The listing builds one solid part. Answer for the finished solid, in the listing's coordinates (mm). A direction names the side the tool comes from. Give positions to 0.01 mm unless a question says otherwise; leave off trailing zeros. Write each loop counter-clockwise with the first axis right and the second up, starting at its lowest first coordinate (ties: lowest second). Pieces come first, ordered by that corner, then holes. Notation, with made-up numbers: (65.25, 71.25) - (73.25, 71.25) arc R22 ccw to (73.25, 97.25) - close; hole circle Ø7 at (-35, 45). An arc over 180 degrees is marked (long way). Use a Markdown table: item, result. Add a question column.
from build123d import *

# Parameters (mm, degrees)
SKETCH1_W           = 12.7
SKETCH1_H           = 25.4
BOSS_EXTRUDE1_DEPTH = 3.175
SKETCH2_W           = 12.7
SKETCH2_H           = 3.175
BOSS_EXTRUDE2_DEPTH = 13.7922
SKETCH3_R           = 2.54
CUT_EXTRUDE1_DEPTH  = 4.175
CUT_EXTRUDE2_DEPTH  = 4.175
SKETCH5_R           = 2.54
CUT_EXTRUDE3_DEPTH  = 4.175
CUT_EXTRUDE4_DEPTH  = 4.175


with BuildPart() as part:
    # Sketch1 → Boss-Extrude1 (new body)
    with BuildSketch(Plane(origin=(0, 0, 0), x_dir=(1, 0, 0), z_dir=(0, 1, 0))):
        with Locations((-19.111794294, -7.819421488)):
            Rectangle(SKETCH1_W, SKETCH1_H)
    extrude(amount=BOSS_EXTRUDE1_DEPTH)

    # Sketch2 → Boss-Extrude2 (add)
    with BuildSketch(Plane(origin=(0, 3.175, 0), x_dir=(1, 0, 0), z_dir=(0, 1, 0))):
        with Locations((-19.111794294, -18.931921488)):
            Rectangle(SKETCH2_W, SKETCH2_H)
    extrude(amount=BOSS_EXTRUDE2_DEPTH)

    # Sketch3 → Cut-Extrude1 (cut, through all)
    with BuildSketch(Plane(origin=(0, 3.175, 0), x_dir=(1, 0, 0), z_dir=(0, 1, 0))):
        with Locations((-19.111794294, -2.739421488)):
            Circle(SKETCH3_R)
    extrude(amount=-CUT_EXTRUDE1_DEPTH, mode=Mode.SUBTRACT)

    # Sketch4 → Cut-Extrude2 (cut, through all)
    with BuildSketch(Plane(origin=(0, 3.175, 0), x_dir=(1, 0, 0), z_dir=(0, 1, 0))):
        with BuildLine():
            Line((-25.461794294, 4.880578512), (-12.761794294, 4.880578512))
            Line((-12.761794294, 4.880578512), (-12.761794294, 1.385127101))
            ThreePointArc((-12.761794294, 1.385127101), (-19.111794294, 4.832526813), (-25.461794294, 1.385127101))
            Line((-25.461794294, 1.385127101), (-25.461794294, 4.880578512))
        make_face()
    extrude(amount=-CUT_EXTRUDE2_DEPTH, mode=Mode.SUBTRACT)

    # Sketch5 → Cut-Extrude3 (cut, through all)
    with BuildSketch(Plane(origin=(0, 0, 17.344421488), x_dir=(-1, 0, 0), z_dir=(0, 0, -1))):
        with Locations((19.111794294, 9.0932)):
            Circle(SKETCH5_R)
    extrude(amount=-CUT_EXTRUDE3_DEPTH, mode=Mode.SUBTRACT)

    # Sketch6 → Cut-Extrude4 (cut, through all)
    with BuildSketch(Plane(origin=(0, 0, 17.344421488), x_dir=(-1, 0, 0), z_dir=(0, 0, -1))):
        with BuildLine():
            Line((25.461794294, 16.9672), (12.761794294, 16.9672))
            Line((12.761794294, 16.9672), (12.761794294, 13.704377903))
            ThreePointArc((12.761794294, 13.704377903), (19.111794294, 16.940840515), (25.461794294, 13.704377903))
            Line((25.461794294, 13.704377903), (25.461794294, 16.9672))
        make_face()
    extrude(amount=-CUT_EXTRUDE4_DEPTH, mode=Mode.SUBTRACT)


solid = part.part
1. Which of the six approach directions +Z, -Z, +X, -X, +Y, -Y give full straight-line access (tool end or side, diameter ignored) to faces 4 (the cylindrical face through (-21.46, 8.12, 18.91)), 5 (the flat face through (-17.8, 11.5, 17.344))?
2. The part is cut by section C-C (x = -20.75). Give the vertices of the cut face in (y, z) (3 decimals), and give its area (3 significant figures).
3. The part is cut by section D-D (z = 6.75). Give the vertices of the cut face in (x, y) (3 decimals).
4. Given P1, Ø4, axis at x = -19.11, y = 9.09, coming from the +Z side; P2, Ø4, axis at x = -16.5, y = 10.5, coming from the -Z side; P3, Ø6.5, axis at x = -18.5, z = 10.5, coming from the +Y side (3 decimals), each flat-ended and moving along its own axis, determine where each tip first touches the part or whether it passes through.
5. Consider L1, parallel to Y at x = -16.5, z = 7.75 (3 decimals); L2, parallel to Z at x = -24.25, y = 5.5; L3, parallel to Z at x = -15.5, y = 1.25. Determine where each line is inside the solid, lowest interval first. Write a range as [from, to].
6. For a pull along Z with two mould halves and no side action, classify faces 1 (the flat face through (-19, 6, 20.519)), 2 (the flat face through (-12.762, 3, 14)), 3 (the cylindrical face through (-16.765, 1.61, 3.712)) as released by +Z, released by -Z, zero draft, split by the parting line, or undercut.
7. The part is cut by section A-A (z = 4). Give the vertices of the cut face in (x, y) (3 decimals), and give its area (3 significant figures).
8. The part is cut by section B-B (y = 10.75). Give the vertices of the cut face in (x, z).
Check values:
| question | item | result |
|---|---|---|
| 1 | face 4 | +Z, -Z |
| 1 | face 5 | -Z, +X, -X, +Y |
| 2 | outline | (0, -4.653) - (3.175, -4.653) - (3.175, 0.798) - (0, 0.798) - close; (0, 4.681) - (3.175, 4.681) - (3.175, 17.344) - (7.152, 17.344) - (7.152, 20.519) - (0, 20.519) - close; (11.034, 17.344) - (16.768, 17.344) - (16.768, 20.519) - (11.034, 20.519) - close |
| 2 | area | 98.4 mm2 |
| 3 | outline | (-25.462, 0) - (-12.762, 0) - (-12.762, 3.175) - (-25.462, 3.175) - close |
| 4 | P1 | passes through |
| 4 | P2 | stops at z = 17.34 |
| 4 | P3 | stops at y = 3.175 |
| 5 | L1 | y = [0, 3.175] |
| 5 | L2 | z = [17.34, 20.52] |
| 5 | L3 | z = [-3.92, 20.52] |
| 6 | face 1 | released by +Z |
| 6 | face 2 | zero draft |
| 6 | face 3 | undercut |
| 7 | outline | (-25.462, 0) - (-21.317, 0) - (-21.317, 3.175) - (-25.462, 3.175) - close; (-16.907, 0) - (-12.762, 0) - (-12.762, 3.175) - (-16.907, 3.175) - close |
| 7 | area | 26.3 mm2 |
| 8 | outline | (-25.46, 17.34) - (-21.04, 17.34) - (-21.04, 20.52) - (-25.46, 20.52) - close; (-17.19, 17.34) - (-12.76, 17.34) - (-12.76, 20.52) - (-17.19, 20.52) - close |
